Read the model definition and answer for the solid it produces. Units are mm, in the model's axes. A direction names the side the tool comes from. Round coordinates to 2 decimals unless told otherwise and drop trailing zeros. Write each loop counter-clockwise with the first axis right and the second up, starting at its lowest first coordinate (ties: lowest second). Pieces come first, ordered by that corner, then holes. Notation, with made-up numbers: (80, 44) - (135, 44) arc R29 cw to (135, 82) - close; hole circle Ø1 at (-8, 63.25). An arc over 180 degrees is marked (long way). Answer as CSV lines item,"result". Start each with the question number.
1) Find section C-C on y = -10. Determine the outline of the cut face in (x, z), then the cut area to 3 significant figures.
2) Which of the six approach directions +Z, -Z, +X, -X, +Y, -Y give full straight-line access (tool end or side, diameter ignored) to faces 1 (the cylindrical face through (-197.685, 78.986, -43.898)), 2 (the cylindrical face through (-89.05, 23.66, 214.77)), 3 (the cylindrical face through (60.075, 38.454, 190.764))?
3) For a pull along Z with two mould halves and no side action, classify faces 4 (the flat face through (53, 0, -225)), 5 (the flat face through (149, 78, 29)), 6 (the cylindrical face through (-91.273, 118.426, -119.035)), 7 (the cylindrical face through (45.356, 119.44, 144.027)) as +Z half, -Z half, draft (parallel to the pull), parting line (faces both ways), or undercut.
4) Consider line 1 along X through (y, z) = (118, 0); line 2 along X through (y, z) = (-15.5, 0); line 3 along Z through (x, y) = (56, -22.5). Determine where each line is inside the solid, lowest interval first.
5) Find section B-B on y = 129. Determine the outline of the cut face in (x, z), then the cut area to 3 significant figures.
6) Each of these flat-tipped pins is pushed along its axis until it touches: pin 1 (1.5 mm diameter, centred on x = -170.5, y = 0.5, fed in from -Z); pin 2 (5 mm diameter, centred on y = 89, z = 96, fed in from +X); pin 3 (12 mm diameter, centred on x = 132, y = 108, fed in from -Z). Where does it stop, or does it pass through?
7) Find section A-A on z = 0. Determine the outline of the cut face in (x, y).
from build123d import *

# Parameters (mm, degrees)
SKETCH_1_R        = 232.5
SKETCH_1_R_2      = 200
EXTRUDE_1_DEPTH   = 78
SKETCH_2_R        = 151
SKETCH_2_R_2      = 150
EXTRUDE_2_DEPTH   = 82
CHAMFER_1_SIZE    = 30
SKETCH_4_R        = 202.5
SKETCH_4_R_2      = 150
EXTRUDE_1_2_DEPTH = 2
SKETCH_5_R        = 230
SKETCH_5_R_2      = 229
EXTRUDE_2_2_DEPTH = 60


with BuildPart() as part:
    # Эскиз1 → Extrude 1 (new body)
    with BuildSketch(Plane(origin=(0, 0, 0), x_dir=(1, 0, 0), z_dir=(0, 1, 0))):
        with Locations(Location((0, 0, 0), (0, 0, 270))):
            Circle(SKETCH_1_R)
        with Locations(Location((0, 0, 0), (0, 0, 270))):
            Circle(SKETCH_1_R_2, mode=Mode.SUBTRACT)
    extrude(amount=EXTRUDE_1_DEPTH)

    # Фаска1
    chamfer_1_edges = [part.edges().sort_by_distance(p)[0] for p in [
        (0, 78, -232.5),
    ]]
    chamfer(chamfer_1_edges, length=CHAMFER_1_SIZE)



with BuildPart() as body_2:
    # Эскиз2 → Extrude 2 (new body)
    with BuildSketch(Plane(origin=(0, 78, 0), x_dir=(1, 0, 0), z_dir=(0, 1, 0))):
        with Locations(Location((0, 0, 0), (0, 0, 270))):
            Circle(SKETCH_2_R)
        with Locations(Location((0, 0, 0), (0, 0, 270))):
            Circle(SKETCH_2_R_2, mode=Mode.SUBTRACT)
    extrude(amount=EXTRUDE_2_DEPTH)


with BuildPart() as part_1:
    add(part.part)

    add(body_2.part)  # Extrude 1 2 merges body 2
    # Эскиз4 → Extrude 1 2 (add)
    with BuildSketch(Plane(origin=(0, 78, 0), x_dir=(1, 0, 0), z_dir=(0, 1, 0))):
        with Locations(Location((0, 0, 0), (0, 0, 270))):
            Circle(SKETCH_4_R)
        with Locations(Location((0, 0, 0), (0, 0, 270))):
            Circle(SKETCH_4_R_2, mode=Mode.SUBTRACT)
    extrude(amount=EXTRUDE_1_2_DEPTH)

    # Эскиз5 → Extrude 2 2 (add)
    with BuildSketch(Plane.XZ):
        with Locations(Location((0, 0, 0), (0, 0, 90))):
            Circle(SKETCH_5_R)
        with Locations(Location((0, 0, 0), (0, 0, 270))):
            Circle(SKETCH_5_R_2, mode=Mode.SUBTRACT)
    extrude(amount=EXTRUDE_2_2_DEPTH)


solid = part_1.part
Check values:
1,outline,"circle Ø460 at (0, 0); hole circle Ø458 at (0, 0)"
1,area,"1,440 mm^2"
2,face 1,"+Y"
2,face 2,"+Y, -Y"
2,face 3,"-Y"
3,face 4,"draft"
3,face 5,"undercut"
3,face 6,"undercut"
3,face 7,"parting line"
4,line 1,"x = -151 to -150, 150 to 151"
4,line 2,"x = -230 to -229, 229 to 230"
4,line 3,"z = -223.08 to -222.05, 222.05 to 223.08"
5,outline,"circle Ø302 at (0, 0); hole circle Ø300 at (0, 0)"
5,area,"946 mm^2"
6,pin 1,"stops at z = -158.87"
6,pin 2,"stops at x = 118.57"
6,pin 3,"stops at z = -83.22"
7,outline,"(-232.5, 0) - (-230, 0) - (-230, -60) - (-229, -60) - (-229, 0) - (-200, 0) - (-200, 78) - (-150, 78) - (-150, 160) - (-151, 160) - (-151, 80) - (-202.5, 80) - (-202.5, 78) - (-232.5, 48) - close; (150, 78) - (200, 78) - (200, 0) - (229, 0) - (229, -60) - (230, -60) - (230, 0) - (232.5, 0) - (232.5, 48) - (202.5, 78) - (202.5, 80) - (151, 80) - (151, 160) - (150, 160) - close"
